Part print with two shaded views. Sizes in mm from the minimum x, y, z corner. A direction names the side the tool comes from. Coordinates: 2 decimals unless noted, no trailing zeros. Write each loop counter-clockwise with the first axis right and the second up, starting at its lowest first coordinate (ties: lowest second). Pieces come first, ordered by that corner, then holes. Notation, with made-up numbers: M 51.25,55.25 L 88.25,55.25 A13 ccw 88.25,71.25 Z; hole C -15,-11.75 d11. An arc over 180 degrees is marked long. One line per question, with ' | ' between items. Start each with the question number.
(1) Tool access for the marked faces 1, 2, 3 and 4: list every direction of +Z, -Z, +X, -X, +Y, -Y with a clear straight run to the whole face (end or side of a thin tool).
(2) Cut at C-C (z = 2.5). Write the cut outline in (x, y).
(3) Wall check: probe 1 along Y at (x, z) = (30, 7); probe 2 along Y at (x, z) = (37, 1); probe 3 along X at (y, z) = (21.5, 9). Give the ranges that are in metal, low to high.
(4) Two-plate mould, pull along Y, no slides. Class the marked faces 5, 6 and 7: +Y half, -Y half, draft (parallel to the pull), parting line (faces both ways), or undercut.
(5) Flat gauge pins, fed straight in: pin 1 Ø4.5 at (x, z) = (4.88, 10.26) entering from -Y; pin 2 Ø3 at (x, y) = (50.5, 12.5) entering from +Z (3 decimals); pin 3 Ø4 at (x, z) = (19, 9.5) entering from +Y; pin 4 Ø12 at (y, z) = (10.5, 11) entering from -X (1 decimal). Where does each tip first touch, or does it go through?
(6) Cut at B-B (y = 35.5). Write the cut outline in (x, z).
(7) Cut at A-A (x = 30). Write the cut outline in (y, z).
(8) Cut at D-D (x = 46). Write the cut outline in (y, z) (1 decimal), plus the area to 3 significant figures.
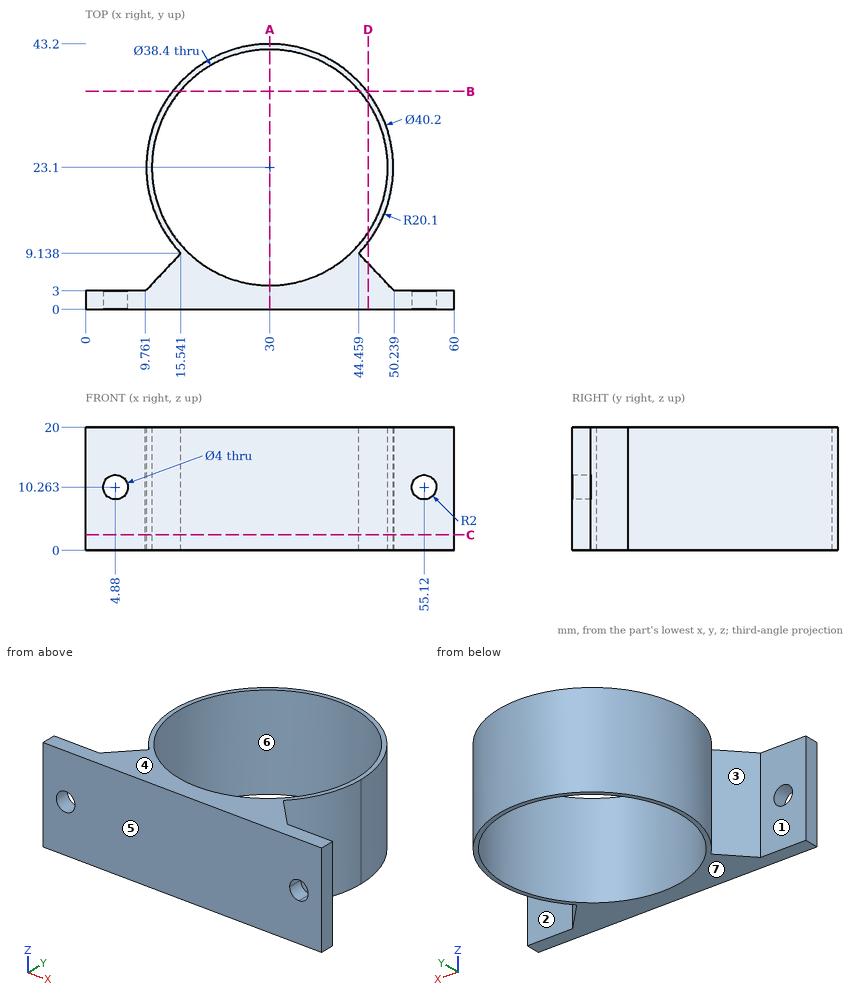
Filled in:
1) face 1: +Z, -Z, -X, +Y | face 2: +Z, -Z, +X, +Y | face 3: +Z, -Z, -X | face 4: +Z, +X, -X, +Y, -Y
2) outline: M 0,0 L 60,0 L 60,3 L 50.24,3 L 44.46,9.14 A20.1 ccw 50.1,23.1 A20.1 ccw long 15.54,9.14 L 9.76,3 L 0,3 Z; hole C 30,23.1 d38.4
3) probe 1: 0 to 3.9, 42.3 to 43.2 | probe 2: 0 to 5.22, 40.98 to 41.94 | probe 3: 9.96 to 10.87, 49.13 to 50.04
4) face 5: -Y half | face 6: undercut | face 7: draft
5) pin 1: y = 0 | pin 2: through | pin 3: y = 41.07 | pin 4: x = 11
6) outline: M 14.18,0 L 15.34,0 L 15.34,20 L 14.18,20 Z; M 44.66,0 L 45.82,0 L 45.82,20 L 44.66,20 Z
7) outline: M 0,0 L 3.9,0 L 3.9,20 L 0,20 Z; M 42.3,0 L 43.2,0 L 43.2,20 L 42.3,20 Z
8) outline: M 0,0 L 7.5,0 L 7.5,20 L 0,20 Z; M 10.9,0 L 12.5,0 L 12.5,20 L 10.9,20 Z; M 33.7,0 L 35.3,0 L 35.3,20 L 33.7,20 Z | area: 212 mm²
